The listing builds one solid part. Answer for the finished solid, in the listing's coordinates (mm). Face numbers are marked on the shaded views. A direction names the side the tool comes from. Coordinates: 2 decimals unless noted, no trailing zeros. Write each loop counter-clockwise with the first axis right and the second up, starting at its lowest first coordinate (ties: lowest second). Pieces come first, ordered by that corner, then holes.
(1) The part is cut by section A-A on z = 1. Determine the outline of the cut face in (x, y).
(2) Which of the six approach directions +Z, -Z, +X, -X, +Y, -Y give full straight-line access (tool end or side, diameter ignored) to the marked faces 1 and 2?
(3) The part is cut by section B-B on y = 18.75. Determine the outline of the cut face in (x, z).
(4) Given P1, Ø16, axis at x = 0, z = 0, coming from the +Y side; P2, Ø3, axis at x = -6.5, z = 3, coming from the -Y side; P3, Ø8, axis at x = 23, y = 17.5, coming from the +Z side, each flat-ended and moving along its own axis, determine where each tip first touches the part or whether it passes through.
(5) The part is cut by section D-D on z = -5. Determine the outline of the cut face in (x, y), plus the area to 3 significant figures.
(6) The part is cut by section C-C on x = 8.5. Determine the outline of the cut face in (y, z), plus the area to 3 significant figures.
(7) For a pull along X with two mould halves and no side action, classify the marked faces 3, 4, 5 and 6 as +X half, -X half, draft (parallel to the pull), parting line (faces both ways), or undercut.
(8) Straight lines are drawn through the part: line 1 (X direction, y = 15.75, z = 0); line 2 (X direction, y = 5.5, z = 0); line 3 (Y direction, x = 6, z = 13.5). For each, find the intervals that lie inside material, in ascending order.
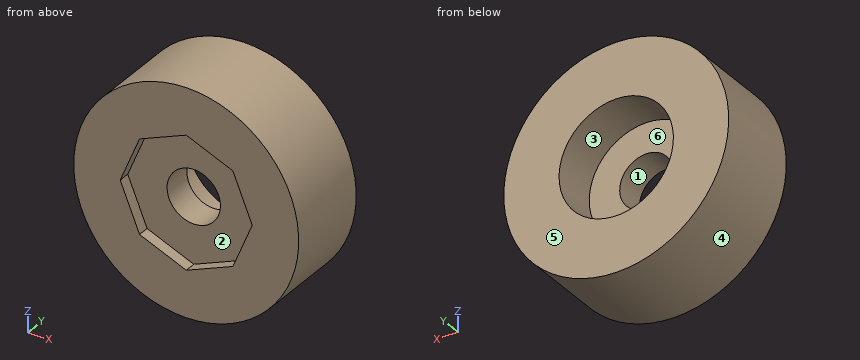
from build123d import *

# Parameters (mm, degrees)
SKETCH1_R           = 29.5
BOSS_EXTRUDE1_DEPTH = 22.9
CUT_EXTRUDE1_DEPTH  = 3
SKETCH3_R           = 7
CUT_EXTRUDE2_DEPTH  = 8
SKETCH4_R           = 15
CUT_EXTRUDE3_DEPTH  = 12


with BuildPart() as part:
    # Sketch1 → Boss-Extrude1 (new body)
    with BuildSketch(Plane(origin=(0, 0, 0), x_dir=(1, 0, 0), z_dir=(0, 1, 0))):
        with Locations(Location((0, 0, 0), (0, 0, 270))):
            Circle(SKETCH1_R)
    extrude(amount=BOSS_EXTRUDE1_DEPTH)

    # Sketch2 → Cut-Extrude1 (cut)
    with BuildSketch(Plane.XZ):
        Polygon((12.245869836, 12.245869836), (0, 17.318275205), (-12.245869836, 12.245869836), (-17.318275205, 0), (-12.245869836, -12.245869836), (0, -17.318275205), (12.245869836, -12.245869836), (17.318275205, 0), align=None)
    extrude(amount=-CUT_EXTRUDE1_DEPTH, mode=Mode.SUBTRACT)

    # Sketch3 → Cut-Extrude2 (cut)
    with BuildSketch(Plane.XZ.offset(-3)):
        with Locations(Location((0, 0, 0), (0, 0, 270))):
            Circle(SKETCH3_R)
    extrude(amount=-CUT_EXTRUDE2_DEPTH, mode=Mode.SUBTRACT)

    # Sketch4 → Cut-Extrude3 (cut)
    with BuildSketch(Plane(origin=(0, 22.9, 0), x_dir=(1, 0, 0), z_dir=(0, 1, 0))):
        with Locations(Location((0, 0, 0), (0, 0, 270))):
            Circle(SKETCH4_R)
    extrude(amount=-CUT_EXTRUDE3_DEPTH, mode=Mode.SUBTRACT)


solid = part.part
Model answer:
1. outline: (-29.48, 0) - (-16.9, 0) - (-16.9, 3) - (-6.93, 3) - (-6.93, 10.9) - (-14.97, 10.9) - (-14.97, 22.9) - (-29.48, 22.9) - close; (6.93, 3) - (16.9, 3) - (16.9, 0) - (29.48, 0) - (29.48, 22.9) - (14.97, 22.9) - (14.97, 10.9) - (6.93, 10.9) - close
2. face 1: +Y, -Y
2. face 2: -Y
3. outline: circle Ø59 at (0, 0); hole circle Ø30 at (0, 0)
4. P1: stops at y = 10.9
4. P2: stops at y = 3
4. P3: stops at z = 22.57
5. outline: (-29.07, 0) - (-15.25, 0) - (-15.25, 3) - (-4.9, 3) - (-4.9, 10.9) - (-14.14, 10.9) - (-14.14, 22.9) - (-29.07, 22.9) - close; (4.9, 3) - (15.25, 3) - (15.25, 0) - (29.07, 0) - (29.07, 22.9) - (14.14, 22.9) - (14.14, 10.9) - (4.9, 10.9) - close
5. area: 823 mm2
6. outline: (0, -28.25) - (22.9, -28.25) - (22.9, -12.36) - (10.9, -12.36) - (10.9, 12.36) - (22.9, 12.36) - (22.9, 28.25) - (0, 28.25) - (0, 13.8) - (3, 13.8) - (3, -13.8) - (0, -13.8) - close
6. area: 914 mm2
7. face 3: undercut
7. face 4: parting line
7. face 5: draft
7. face 6: undercut
8. line 1: x = -29.5 to -15, 15 to 29.5
8. line 2: x = -29.5 to -7, 7 to 29.5
8. line 3: y = 3 to 10.9
